Part model, mm, in its own coordinate system. A direction names the side the tool comes from. Coordinates: 2 decimals unless noted, no trailing zeros. Loops run counter-clockwise (first coordinate to the right, second up) from the corner with the lowest first, then second, coordinate; pieces in that order, holes last. Notation, with made-up numbers: (-0.75, 3.5) - (34.25, 3.5) arc R18 ccw to (34.25, 31.5) - close; hole circle Ø8 at (-7, 70). An arc over 180 degrees is marked (long way). Use a Markdown table: item, result. Add a question column.
1. Band-saw the part on A-A, the plane x = 22.5. Give the cut face in (y, z), plus the area to 3 significant figures.
2. Wall check: probe 1 along Y at (x, z) = (52, -44); probe 2 along X at (y, z) = (3.5, -4); probe 3 along Z at (x, y) = (87.5, -2.25). Give the ranges that are in metal, low to high. Write a range as [from, to].
3. Band-saw the part on B-B, the plane z = -32.5. Give the cut face in (x, y), plus the area to 3 significant figures.
4. Drop flat-ended pins along their axis: pin 1 (3.5 mm diameter, centred on y = -0.5, z = 19, fed in from +X); pin 2 (1.6 mm diameter, centred on x = 94.5, y = -1, fed in from -Z); pin 3 (0.6 mm diameter, centred on x = 95, y = -0.5, fed in from +Z). Give the stop position or say it passes through.
5. 3-axis set-ups, long thin cutter, end or side, ignore diameter. For faces 1 (the cylindrical face through (92.65, -0.07, 54.99)), 2 (the cylindrical face through (88.105, -1.609, 20.177)), 3 (the flat face through (0, -4, 1)): which of +Z, -Z, +X, -X, +Y, -Y reach the whole face in a straight line?
6. Pull direction Y, two halves, no side cores. Call faces 4 (the flat face through (80.5, -1, 18)), 5 (the flat face through (93.5, -1, 6)), 6 (the flat face through (86, -4, 50)), 7 (the flat face through (-1, 5, 1)): pulls with the +Y half, pulls with the -Y half, needs draft (parallel to the pull), parting line crosses it, or undercut.
from build123d import *

# Parameters (mm, degrees)
F1_DEPTH  = 5
F2_W      = 156.496823
F2_H      = 91.289811
F2_R      = 2.986594
F3_DEPTH  = 1
F4_DEPTH  = 1
F6_DEPTH  = 1
F7_R      = 2.053092
F8_DEPTH  = 15
F9_W      = 4.116406
F9_H      = 9.901583
F10_DEPTH = 2
F11_W     = 4.423767
F11_H     = 9.900813
F12_DEPTH = 2


with BuildPart() as f1:
    # F0 (on Front) → F1 (new body, symmetric)
    with BuildSketch(Plane.XZ):
        with BuildLine():
            Line((85.5, 58), (-85.5, 58))
            ThreePointArc((-85.5, 58), (-92.571068, 55.071068), (-95.5, 48))
            Line((-95.5, 48), (-95.5, -48))
            ThreePointArc((-95.5, -48), (-92.571068, -55.071068), (-85.5, -58))
            Line((-85.5, -58), (85.5, -58))
            ThreePointArc((85.5, -58), (92.571068, -55.071068), (95.5, -48))
            Line((95.5, -48), (95.5, 48))
            ThreePointArc((95.5, 48), (92.571068, 55.071068), (85.5, 58))
        make_face()
    extrude(amount=F1_DEPTH, both=True)

    # F2 (on face) → F3 (cut)
    with BuildSketch(Plane.XZ.offset(5)):
        with Locations((0.742533, 0.334394)):
            Rectangle(F2_W, F2_H)
        with Locations((86.493112, 50.336968)):
            Circle(F2_R)
    extrude(amount=-F3_DEPTH, mode=Mode.SUBTRACT)

    # F2 (on face) → F4 (cut)
    with BuildSketch(Plane.XZ.offset(5)):
        with Locations((0.742533, 0.334394)):
            Rectangle(F2_W, F2_H)
        with Locations((86.493112, 50.336968)):
            Circle(F2_R)
    extrude(amount=-F4_DEPTH, mode=Mode.SUBTRACT)

    # F5 (on face) → F6 (join)
    with BuildSketch(Plane.YZ.offset(95.5)):
        with BuildLine():
            Line((-0.305085, 35.823516), (-1.833566, 35.823516))
            ThreePointArc((-1.833566, 35.823516), (-2.540673, 35.530623), (-2.833566, 34.823516))
            Line((-2.833566, 34.823516), (-2.833566, 26.449343))
            ThreePointArc((-2.833566, 26.449343), (-2.540673, 25.742236), (-1.833566, 25.449343))
            Line((-1.833566, 25.449343), (-0.305085, 25.449343))
            ThreePointArc((-0.305085, 25.449343), (0.402022, 25.742236), (0.694915, 26.449343))
            Line((0.694915, 26.449343), (0.694915, 34.823516))
            ThreePointArc((0.694915, 34.823516), (0.402022, 35.530623), (-0.305085, 35.823516))
        make_face()
    extrude(amount=F6_DEPTH)

    # F7 (on face) → F8 (cut)
    with BuildSketch(Plane.YZ.offset(95.5)):
        with Locations((-1.342217, 18.141782)):
            Circle(F7_R)
    extrude(amount=-F8_DEPTH, mode=Mode.SUBTRACT)

    # F9 (on face) → F10 (cut)
    with BuildSketch(Plane.YZ.offset(95.5)):
        with Locations((-1.26129, 6.061323)):
            Rectangle(F9_W, F9_H)
    extrude(amount=F10_DEPTH, mode=Mode.SUBTRACT)

    # F11 (on face) → F12 (cut)
    with BuildSketch(Plane.YZ.offset(95.5)):
        with Locations((-1.390659, 6.107518)):
            Rectangle(F11_W, F11_H)
    extrude(amount=-F12_DEPTH, mode=Mode.SUBTRACT)


solid = f1.part
Geometry check:
| question | item | result |
|---|---|---|
| 1 | outline | (-5, -58) - (5, -58) - (5, 58) - (-5, 58) - (-5, 45.98) - (-4, 45.98) - (-4, -45.31) - (-5, -45.31) - close |
| 1 | area | 1,070 mm^2 |
| 2 | probe 1 | y = [-4, 5] |
| 2 | probe 2 | x = [-95.5, 95.5] |
| 2 | probe 3 | z = [-57.8, 16.3], [19.98, 57.8] |
| 3 | outline | (-95.5, -5) - (-77.51, -5) - (-77.51, -4) - (78.99, -4) - (78.99, -5) - (95.5, -5) - (95.5, 5) - (-95.5, 5) - close |
| 3 | area | 1,750 mm^2 |
| 4 | pin 1 | stops at x = 95.5 |
| 4 | pin 2 | stops at z = -53.72 |
| 4 | pin 3 | stops at z = 51.92 |
| 5 | face 1 | +Z, +X, +Y, -Y |
| 5 | face 2 | +X |
| 5 | face 3 | -Y |
| 6 | face 4 | undercut |
| 6 | face 5 | undercut |
| 6 | face 6 | pulls with the -Y half |
| 6 | face 7 | pulls with the +Y half |
